Autodesk Inventor part; units mm, degrees
ref_plane "YZ Plane" through (0, 0, 0) normal (1, 0, 0) x (0, 1, 0)
ref_plane "XZ Plane" through (0, 0, 0) normal (0, 1, 0) x (-1, 0, 0)
ref_plane "XY Plane" through (0, 0, 0) normal (0, 0, 1) x (1, 0, 0)
sketch "Esboço1" plane through (0, 0, 0) normal (1, 0, 0) x (0, 1, 0)
  line L0 (-121, -21) -> (121, -21)
  line L1 (121, -21) -> (121, 21)
  line L2 (121, 21) -> (-121, 21)
  line L3 (-121, 21) -> (-121, -21)
  line L4 (-121, -21) -> (121, 21) construction
  line L5 (121, -21) -> (-121, 21) construction
  line L6 (-121, 21) -> (-79, 21) construction
  line L7 (-79, 21) -> (-79, -21) construction
  line L8 (-79, -21) -> (-121, -21) construction
  line L9 (-121, -21) -> (-121, 21) construction
  line L10 (-115.5, -15.5) -> (-84.5, -15.5) construction
  line L11 (-84.5, -15.5) -> (-84.5, 15.5) construction
  line L12 (-84.5, 15.5) -> (-115.5, 15.5) construction
  line L13 (-115.5, 15.5) -> (-115.5, -15.5) construction
  line L14 (-115.5, -15.5) -> (-84.5, 15.5) construction
  line L15 (-84.5, -15.5) -> (-115.5, 15.5) construction
  circle A0 centre (-100, 0) radius 11.5
  line L16 (-25, 0) -> (25, 0) construction
  line L17 (-17.5, -7.5) -> (17.5, -7.5)
  line L18 (17.5, 7.5) -> (-17.5, 7.5)
  arc A1 (-17.5, 7.5) -> (-17.5, -7.5) centre (-17.5, 0) ccw
  arc A2 (17.5, -7.5) -> (17.5, 7.5) centre (17.5, 0) ccw
  line L19 (-79, 15) -> (-68.8, 15)
  line L20 (-68.8, 15) -> (-68.8, 12)
  line L21 (-68.8, 12) -> (-79, 12)
  line L22 (-79, 12) -> (-79, 15)
  line L23 (-25.2, 15) -> (-15, 15)
  line L24 (-15, 15) -> (-15, 12)
  line L25 (-15, 12) -> (-25.2, 12)
  line L26 (-25.2, 12) -> (-25.2, 15)
  circle A3 centre (-58.8, 13.5) radius 5 construction
  line L27 (-121, 0) -> (121, 0) construction
  line L28 (-79, -15) -> (-68.8, -15)
  line L29 (-68.8, -15) -> (-68.8, -12)
  line L30 (-68.8, -12) -> (-79, -12)
  line L31 (-79, -12) -> (-79, -15)
  line L32 (-25.2, -15) -> (-15, -15)
  line L33 (-15, -15) -> (-15, -12)
  line L34 (-15, -12) -> (-25.2, -12)
  line L35 (-25.2, -12) -> (-25.2, -15)
  circle A4 centre (-58.8, -13.5) radius 5 construction
  line L36 (0, -21) -> (0, 21) construction
  circle A5 centre (100, 0) radius 11.5
  line L37 (79, 15) -> (68.8, 15)
  line L38 (68.8, 15) -> (68.8, 12)
  line L39 (68.8, 12) -> (79, 12)
  line L40 (79, 12) -> (79, 15)
  line L41 (25.2, 15) -> (15, 15)
  line L42 (15, 15) -> (15, 12)
  line L43 (15, 12) -> (25.2, 12)
  line L44 (25.2, 12) -> (25.2, 15)
  line L45 (68.8, -15) -> (68.8, -12)
  line L46 (79, -15) -> (68.8, -15)
  line L47 (79, -12) -> (79, -15)
  line L48 (68.8, -12) -> (79, -12)
  line L49 (25.2, -12) -> (25.2, -15)
  line L50 (25.2, -15) -> (15, -15)
  line L51 (15, -12) -> (25.2, -12)
  line L52 (15, -15) -> (15, -12)
  point P0 (0, 0)
  point P1 (-100, 0)
  point P2 (-100, 21)
  point P3 (0, 0)
  point P4 (0, 0)
  point P5 (-68.8, 13.5)
  point P6 (-68.8, -13.5)
  point P7 (68.8, 13.5)
  point P8 (68.8, -13.5)
  dimension "d0" = 242
  dimension "d1" = 42
  dimension "d2" = 42
  dimension "d3" = 42
  dimension "d4" = 31
  dimension "d5" = 31
  dimension "d6" = 23
  dimension "d7" = 15
  dimension "d8" = 35
  dimension "d9" = 10.2
  dimension "d10" = 3
  dimension "d12" = 6
  dimension "d13" = 10.2
  dimension "d14" = 3
  dimension "d15" = 15
  dimension "d16" = 10
  dimension "d17" = 10
extrude "Extrusão1" add sketch "Esboço1" along normal blind 3
hole "Furo1" at (0, -58.8, 13.5) at (0, -58.8, -13.5) at (0, -84.5, 15.5) at (0, -115.5, 15.5) at (0, -115.5, -15.5) at (0, -84.5, -15.5) direction (1, 0, 0) diameter 3 end through all
mirror "Espelhamento1" about plane through (0, 0, 0) normal (0, 1, 0) of "Furo1"
equation "\"d13\" = d9"
equation "\"d14\" = d10"
properties part number "Lateral_Acrilico"
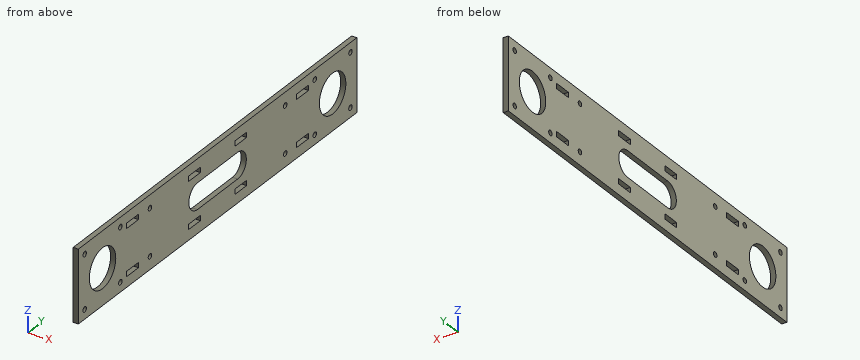
For this review, take the finished solid that the model builds, in its own axes (mm). Coordinates: 2 decimals unless noted, no trailing zeros. Order: outer loops, then holes, each group sorted by start corner. A loop starts at its lowest first (then second) coordinate and runs counter-clockwise, first axis right, second up. Notation, with made-up numbers: (31, 35) - (55, 35) arc R28 cw to (55, 57) - close; hole circle Ø4 at (81.5, 70). An arc over 180 degrees is marked (long way). Use one line per item in the form item = value.
Q1. Consider section D-D (y = -8). Give the boundary of the cut face in (x, z).
Checked values:
outline = (0, -21) - (3, -21) - (3, -7.5) - (0, -7.5) - close; (0, 7.5) - (3, 7.5) - (3, 21) - (0, 21) - close
Q2. Consider section B-B (z = 3). Give the boundary of the cut face in (x, y), then the cut area to 3 significant figures.
Checked values:
outline = (0, -121) - (3, -121) - (3, -111.1) - (0, -111.1) - close; (0, -88.9) - (3, -88.9) - (3, -24.37) - (0, -24.37) - close; (0, 24.37) - (3, 24.37) - (3, 88.9) - (0, 88.9) - close; (0, 111.1) - (3, 111.1) - (3, 121) - (0, 121) - close
area = 447 mm2
Q3. Consider section C-C (x = 2.35). Give the number of separate pieces and of enclosed holes in the cut face, then the cut area to 3 significant figures.
Checked values:
separate_pieces = 1
enclosed_holes = 23
area = 8,300 mm2
Q4. For P1, Ø3.5, axis at y = 115.5, z = 15.5, coming from the +X side, flat-tipped, find the tip position at first contact; note if it passes through.
Checked values:
P1 = 3
Q5. Consider section A-A (y = -100). Give the boundary of the cut face in (x, z), then the cut area to 3 significant figures.
Checked values:
outline = (0, -21) - (3, -21) - (3, -11.5) - (0, -11.5) - close; (0, 11.5) - (3, 11.5) - (3, 21) - (0, 21) - close
area = 57.0 mm2
Q6. For probe 1 along Y at (x, z) = (1.15, 15.5); probe 2 along Z at (x, y) = (1.9, 77.5); probe 3 along Z at (x, y) = (1.2, -84.5), list the stretches that pass through material, from the lowest coordinate up. Write a range as from..to.
Checked values:
probe_1 = -121..-117, -114..-86, -83..83, 86..114, 117..121
probe_2 = -21..-15, -12..12, 15..21
probe_3 = -21..-17, -14..14, 17..21
